```python
from build123d import *

# Parameters (mm, degrees)
SKETCH2_R           = 31.83
BOSS_EXTRUDE1_DEPTH = 8
FILLET1_R           = 2
SKETCH3_R           = 0.5
CUT_EXTRUDE1_DEPTH  = 9


with BuildPart() as part:
    # Sketch2 → Boss-Extrude1 (new body)
    with BuildSketch(Plane.XY):
        with Locations((0, 35.388213047)):
            Circle(SKETCH2_R)
    extrude(amount=BOSS_EXTRUDE1_DEPTH)

    # Fillet1
    fillet1_edges = [part.edges().sort_by_distance(p)[0] for p in [
        (-31.83, 35.388213047, 0),
    ]]
    fillet(fillet1_edges, radius=FILLET1_R)

    # Sketch3 → Cut-Extrude1 (cut, through all)
    with BuildSketch(Plane.XY.offset(8)):
        with Locations((0, 26.458213047)):
            Circle(SKETCH3_R)
    extrude(amount=-CUT_EXTRUDE1_DEPTH, mode=Mode.SUBTRACT)


solid = part.part
```
CAD build for the part. Positions are in the model's coordinates, mm. Coordinates: 2 decimals unless noted, no trailing zeros. Order: outer loops, then holes, each group sorted by start corner. A loop starts at its lowest first (then second) coordinate and runs counter-clockwise, first axis right, second up. Notation, with made-up numbers: (-5, 89.25) - (37, 89.25) arc R25 ccw to (37, 101.25) - close; hole circle Ø11 at (86.5, -31). An arc over 180 degrees is marked (long way). Answer in a Markdown table with one row per item.
1. Flat gauge pins, fed straight in: P1, Ø1.5, axis at y = 10.5, z = 3, coming from the +X side; P2, Ø1.5, axis at y = 51, z = 6.5, coming from the -X side; P3, Ø3, axis at y = 17, z = 2.5, coming from the +X side. Where does each tip first touch, or does it go through?
Answer:
| item | result |
|---|---|
| P1 | x = 20.75 |
| P2 | x = -28.15 |
| P3 | x = 26.98 |
2. Slice it at A-A, the plane z = 2.75. List the corners of the cut face in (x, y).
Answer:
| item | result |
|---|---|
| outline | circle Ø63.66 at (0, 35.39); hole circle Ø1 at (0, 26.46) |
3. Drill centre lines: L1, parallel to Y at x = 0, z = 6; L2, parallel to Y at x = -16, z = 5.5; L3, parallel to X at y = 60.5, z = 1.5. Where is each one in solid material? Low to high. Write a range as from..to.
Answer:
| item | result |
|---|---|
| L1 | 3.56..25.96, 26.96..67.22 |
| L2 | 7.87..62.9 |
| L3 | -19.46..19.46 |
4. Pull direction X, two halves, no side cores. Call faces 1 (the face through (0, 36, 8)), 2 (the face through (-4.144, 66.947, 4.958)): +X half, -X half, draft (parallel to the pull), parting line (faces both ways), or undercut.
Answer:
| item | result |
|---|---|
| face 1 | draft |
| face 2 | parting line |
